from build123d import *

# Parameters (mm, degrees)
SKETCH1_W               = 75
SKETCH1_H               = 90
SKETCH1_W_2             = 50
SKETCH1_H_2             = 13
BOSS_EXTRUDE1_DEPTH     = 8
SKETCH2_R               = 18
SKETCH2_R_2             = 16
BOSS_EXTRUDE2_DEPTH     = 5
SKETCH3_R               = 2
CUT_EXTRUDE2_DEPTH      = 6
CUT_EXTRUDE2_DEPTH_BACK = 9
FILLET2_R               = 10
FILLET3_R               = 10
FILLET4_R               = 10
CUT_EXTRUDE3_REACH      = 10
SKETCH5_R               = 2.5
SKETCH7_W               = 5
SKETCH7_H               = 34
BOSS_EXTRUDE3_DEPTH     = 63
FILLET5_R               = 5
FILLET6_R               = 5
FILLET7_R               = 5
CUT_EXTRUDE4_REACH      = 92
CUT_EXTRUDE5_REACH      = 44
SKETCH14_R              = 2.5
SKETCH14_R_2            = 4


with BuildPart() as part:
    # Sketch1 → Boss-Extrude1 (new body)
    with BuildSketch(Plane(origin=(0, 0, 0), x_dir=(1, 0, 0), z_dir=(0, 1, 0))):
        with Locations((37.5, -45)):
            Rectangle(SKETCH1_W, SKETCH1_H)
        with Locations((100, -83.5)):
            Rectangle(SKETCH1_W_2, SKETCH1_H_2)
    extrude(amount=BOSS_EXTRUDE1_DEPTH)

    # Sketch2 → Boss-Extrude2 (add)
    with BuildSketch(Plane.XZ):
        with Locations((37.5, 45)):
            Circle(SKETCH2_R)
        with Locations((37.5, 45)):
            Circle(SKETCH2_R_2, mode=Mode.SUBTRACT)
    extrude(amount=BOSS_EXTRUDE2_DEPTH)

    # Sketch3 → Cut-Extrude2 (cut, two sides)
    with BuildSketch(Plane.XZ) as cut_extrude2_sk:
        with Locations((8.5, 74)):
            Circle(SKETCH3_R)
        with Locations((66.5, 74)):
            Circle(SKETCH3_R)
        with Locations((8.5, 16)):
            Circle(SKETCH3_R)
        with Locations((66.5, 16)):
            Circle(SKETCH3_R)
    extrude(amount=CUT_EXTRUDE2_DEPTH, mode=Mode.SUBTRACT)
    extrude(cut_extrude2_sk.sketch, amount=-CUT_EXTRUDE2_DEPTH_BACK, mode=Mode.SUBTRACT)

    # Fillet2
    fillet2_edges = [part.edges().sort_by_distance(p)[0] for p in [
        (0, 4, 0),
    ]]
    fillet(fillet2_edges, radius=FILLET2_R)

    # Fillet3
    fillet3_edges = [part.edges().sort_by_distance(p)[0] for p in [
        (0, 4, 90),
    ]]
    fillet(fillet3_edges, radius=FILLET3_R)

    # Fillet4
    fillet4_edges = [part.edges().sort_by_distance(p)[0] for p in [
        (75, 4, 0),
    ]]
    fillet(fillet4_edges, radius=FILLET4_R)

    # Sketch5 → Cut-Extrude3 (cut, up to next)
    with BuildSketch(Plane.XZ, mode=Mode.PRIVATE) as cut_extrude3_sk1:
        with Locations((55, 6)):
            Circle(SKETCH5_R)
    cut_extrude3_tool1 = extrude(cut_extrude3_sk1.sketch, amount=-CUT_EXTRUDE3_REACH, mode=Mode.PRIVATE) & part.part
    add(cut_extrude3_tool1.solids().sort_by_distance((55, 0, 6))[0], mode=Mode.SUBTRACT)
    # Sketch5 → Cut-Extrude3 (cut, up to next)
    with BuildSketch(Plane.XZ, mode=Mode.PRIVATE) as cut_extrude3_sk2:
        with Locations((20, 84)):
            Circle(SKETCH5_R)
    cut_extrude3_tool2 = extrude(cut_extrude3_sk2.sketch, amount=-CUT_EXTRUDE3_REACH, mode=Mode.PRIVATE) & part.part
    add(cut_extrude3_tool2.solids().sort_by_distance((20, 0, 84))[0], mode=Mode.SUBTRACT)
    # Sketch5 → Cut-Extrude3 (cut, up to next)
    with BuildSketch(Plane.XZ, mode=Mode.PRIVATE) as cut_extrude3_sk3:
        with Locations((55, 84)):
            Circle(SKETCH5_R)
    cut_extrude3_tool3 = extrude(cut_extrude3_sk3.sketch, amount=-CUT_EXTRUDE3_REACH, mode=Mode.PRIVATE) & part.part
    add(cut_extrude3_tool3.solids().sort_by_distance((55, 0, 84))[0], mode=Mode.SUBTRACT)
    # Sketch5 → Cut-Extrude3 (cut, up to next)
    with BuildSketch(Plane.XZ, mode=Mode.PRIVATE) as cut_extrude3_sk4:
        with Locations((20, 6)):
            Circle(SKETCH5_R)
    cut_extrude3_tool4 = extrude(cut_extrude3_sk4.sketch, amount=-CUT_EXTRUDE3_REACH, mode=Mode.PRIVATE) & part.part
    add(cut_extrude3_tool4.solids().sort_by_distance((20, 0, 6))[0], mode=Mode.SUBTRACT)

    # Sketch7 → Boss-Extrude3 (add)
    with BuildSketch(Plane(origin=(125, 0, 0), x_dir=(0, 0, -1), z_dir=(1, 0, 0))):
        with Locations((-87.5, 25)):
            Rectangle(SKETCH7_W, SKETCH7_H)
    extrude(amount=-BOSS_EXTRUDE3_DEPTH)

    # Fillet5
    fillet5_edges = [part.edges().sort_by_distance(p)[0] for p in [
        (125, 42, 87.5),
    ]]
    fillet(fillet5_edges, radius=FILLET5_R)

    # Fillet6
    fillet6_edges = [part.edges().sort_by_distance(p)[0] for p in [
        (125, 4, 77),
    ]]
    fillet(fillet6_edges, radius=FILLET6_R)

    # Fillet7
    fillet7_edges = [part.edges().sort_by_distance(p)[0] for p in [
        (62, 42, 87.5),
    ]]
    fillet(fillet7_edges, radius=FILLET7_R)

    # Sketch12 → Cut-Extrude4 (cut, up to next)
    with BuildSketch(Plane.XY.offset(90), mode=Mode.PRIVATE) as cut_extrude4_sk1:
        with BuildLine():
            Line((77.5, 26.5), (87.5, 26.5))
            ThreePointArc((87.5, 26.5), (91.5, 22.5), (87.5, 18.5))
            Line((87.5, 18.5), (77.5, 18.5))
            ThreePointArc((77.5, 18.5), (73.5, 22.5), (77.5, 26.5))
        make_face()
    cut_extrude4_tool1 = extrude(cut_extrude4_sk1.sketch, amount=-CUT_EXTRUDE4_REACH, mode=Mode.PRIVATE) & part.part
    add(cut_extrude4_tool1.solids().sort_by_distance((82.5, 22.5, 90))[0], mode=Mode.SUBTRACT)
    # Sketch12 → Cut-Extrude4 (cut, up to next)
    with BuildSketch(Plane.XY.offset(90), mode=Mode.PRIVATE) as cut_extrude4_sk2:
        with BuildLine():
            Line((70.5, 33), (79.5, 33))
            ThreePointArc((79.5, 33), (81, 31.5), (79.5, 30))
            Line((79.5, 30), (70.5, 30))
            ThreePointArc((70.5, 30), (69, 31.5), (70.5, 33))
        make_face()
    cut_extrude4_tool2 = extrude(cut_extrude4_sk2.sketch, amount=-CUT_EXTRUDE4_REACH, mode=Mode.PRIVATE) & part.part
    add(cut_extrude4_tool2.solids().sort_by_distance((75, 31.5, 90))[0], mode=Mode.SUBTRACT)
    # Sketch12 → Cut-Extrude4 (cut, up to next)
    with BuildSketch(Plane.XY.offset(90), mode=Mode.PRIVATE) as cut_extrude4_sk3:
        with BuildLine():
            Line((70.5, 12), (79.5, 12))
            ThreePointArc((79.5, 12), (81, 13.5), (79.5, 15))
            Line((79.5, 15), (70.5, 15))
            ThreePointArc((70.5, 15), (69, 13.5), (70.5, 12))
        make_face()
    cut_extrude4_tool3 = extrude(cut_extrude4_sk3.sketch, amount=-CUT_EXTRUDE4_REACH, mode=Mode.PRIVATE) & part.part
    add(cut_extrude4_tool3.solids().sort_by_distance((75, 13.5, 90))[0], mode=Mode.SUBTRACT)
    # Sketch12 → Cut-Extrude4 (cut, up to next)
    with BuildSketch(Plane.XY.offset(90), mode=Mode.PRIVATE) as cut_extrude4_sk4:
        with BuildLine():
            Line((103.5, 33), (112.5, 33))
            ThreePointArc((112.5, 33), (114, 31.5), (112.5, 30))
            Line((112.5, 30), (103.5, 30))
            ThreePointArc((103.5, 30), (102, 31.5), (103.5, 33))
        make_face()
    cut_extrude4_tool4 = extrude(cut_extrude4_sk4.sketch, amount=-CUT_EXTRUDE4_REACH, mode=Mode.PRIVATE) & part.part
    add(cut_extrude4_tool4.solids().sort_by_distance((108, 31.5, 90))[0], mode=Mode.SUBTRACT)
    # Sketch12 → Cut-Extrude4 (cut, up to next)
    with BuildSketch(Plane.XY.offset(90), mode=Mode.PRIVATE) as cut_extrude4_sk5:
        with BuildLine():
            Line((103.5, 12), (112.5, 12))
            ThreePointArc((112.5, 12), (114, 13.5), (112.5, 15))
            Line((112.5, 15), (103.5, 15))
            ThreePointArc((103.5, 15), (102, 13.5), (103.5, 12))
        make_face()
    cut_extrude4_tool5 = extrude(cut_extrude4_sk5.sketch, amount=-CUT_EXTRUDE4_REACH, mode=Mode.PRIVATE) & part.part
    add(cut_extrude4_tool5.solids().sort_by_distance((108, 13.5, 90))[0], mode=Mode.SUBTRACT)

    # Sketch14 → Cut-Extrude5 (cut, up to next)
    with BuildSketch(Plane.XZ, mode=Mode.PRIVATE) as cut_extrude5_sk1:
        with Locations((37.5, 57)):
            Circle(SKETCH14_R)
    cut_extrude5_tool1 = extrude(cut_extrude5_sk1.sketch, amount=-CUT_EXTRUDE5_REACH, mode=Mode.PRIVATE) & part.part
    add(cut_extrude5_tool1.solids().sort_by_distance((37.5, 0, 57))[0], mode=Mode.SUBTRACT)
    # Sketch14 → Cut-Extrude5 (cut, up to next)
    with BuildSketch(Plane.XZ, mode=Mode.PRIVATE) as cut_extrude5_sk2:
        with Locations((37.5, 45)):
            Circle(SKETCH14_R_2)
    cut_extrude5_tool2 = extrude(cut_extrude5_sk2.sketch, amount=-CUT_EXTRUDE5_REACH, mode=Mode.PRIVATE) & part.part
    add(cut_extrude5_tool2.solids().sort_by_distance((37.5, 0, 45))[0], mode=Mode.SUBTRACT)
    # Sketch14 → Cut-Extrude5 (cut, up to next)
    with BuildSketch(Plane.XZ, mode=Mode.PRIVATE) as cut_extrude5_sk3:
        with Locations((49.5, 45)):
            Circle(SKETCH14_R)
    cut_extrude5_tool3 = extrude(cut_extrude5_sk3.sketch, amount=-CUT_EXTRUDE5_REACH, mode=Mode.PRIVATE) & part.part
    add(cut_extrude5_tool3.solids().sort_by_distance((49.5, 0, 45))[0], mode=Mode.SUBTRACT)
    # Sketch14 → Cut-Extrude5 (cut, up to next)
    with BuildSketch(Plane.XZ, mode=Mode.PRIVATE) as cut_extrude5_sk4:
        with Locations((37.5, 33)):
            Circle(SKETCH14_R)
    cut_extrude5_tool4 = extrude(cut_extrude5_sk4.sketch, amount=-CUT_EXTRUDE5_REACH, mode=Mode.PRIVATE) & part.part
    add(cut_extrude5_tool4.solids().sort_by_distance((37.5, 0, 33))[0], mode=Mode.SUBTRACT)
    # Sketch14 → Cut-Extrude5 (cut, up to next)
    with BuildSketch(Plane.XZ, mode=Mode.PRIVATE) as cut_extrude5_sk5:
        with Locations((25.5, 45)):
            Circle(SKETCH14_R)
    cut_extrude5_tool5 = extrude(cut_extrude5_sk5.sketch, amount=-CUT_EXTRUDE5_REACH, mode=Mode.PRIVATE) & part.part
    add(cut_extrude5_tool5.solids().sort_by_distance((25.5, 0, 45))[0], mode=Mode.SUBTRACT)


solid = part.part
Here's how the part is built. I have some questions about the finished solid (model axes, mm). A direction names the side the tool comes from. Coordinates: 2 decimals unless noted, no trailing zeros. Loops run counter-clockwise (first coordinate to the right, second up) from the corner with the lowest first, then second, coordinate; pieces in that order, holes last. Notation, with made-up numbers: (-10, 47) -> (22, 47) arc R25 ccw to (22, 59) -> close; hole circle Ø2 at (87, -4.5). An arc over 180 degrees is marked (long way). Use one line per item in the form item = value. Start each with the question number.
(1) If we section it at B-B (x = 109.5): Please give me the cut outline in (y, z), then the cut area to 3 significant figures.
(2) If we section it at D-D (y = 4): Give the number of separate pieces and of enclosed holes in the cut face, then the cut area to 3 significant figures.
(3) Please list where these lines run through material, in increasing order: line 1 along Z through (x, y) = (66, 2); line 2 along Z through (x, y) = (66.5, 4.5); line 3 along Y through (x, z) = (66.5, 57).
(4) If we section it at A-A (z = 45): Please give me the cut outline in (x, y), then the cut area to 3 significant figures.
(5) On a 3-axis mill with a long thin cutter (end or side, diameter ignored), from which of +Z, -Z, +X, -X, +Y, -Y can I reach the whole of each face in a straight line? I mean faces 5 (the face through (66.24, 3.944, 17.983)), 6 (the face through (97, 4, 77)), 7 (the face through (83, 18.5, 88)), 8 (the face through (54.669, -2.465, 50.407)). Say none if no direction works.
(6) We'd pull the mould along Y, two halves only. Please class faces 1 (the face through (34, 0, 64)), 2 (the face through (114, 31.5, 87.5)), 3 (the face through (39, 4, 35)), 4 (the face through (108, 33, 88)): pulls with the +Y half, pulls with the -Y half, needs draft (parallel to the pull), parting line crosses it, or undercut.
(7) If we section it at C-C (y = 22.5): Please give me the cut outline in (x, z).
(8) Will these pins go through, and if not, where does the flat tip stop? pin 1 (8 mm diameter, centred on x = 40.5, z = 62, fed in from +Y); pin 2 (5 mm diameter, centred on x = 66.5, z = 16, fed in from -Y).
Verdict:
q1.outline = (0, 77) -> (8, 77) -> (8, 85) -> (12, 85) -> (12, 90) -> (0, 90) -> close; (15, 85) -> (30, 85) -> (30, 90) -> (15, 90) -> close; (33, 85) -> (42, 85) -> (42, 90) -> (33, 90) -> close
q1.area = 244 mm²
q2.separate_pieces = 1
q2.enclosed_holes = 13
q2.area = 7,070 mm²
q3.line_1 = 0.05 to 14.06, 17.94 to 72.06, 75.94 to 90
q3.line_2 = 0.11 to 14, 18 to 72, 76 to 90
q3.line_3 = 0 to 8
q4.outline = (0, 0) -> (19.5, 0) -> (19.5, -5) -> (21.5, -5) -> (21.5, 0) -> (23, 0) -> (23, 8) -> (0, 8) -> close; (28, 0) -> (33.5, 0) -> (33.5, 8) -> (28, 8) -> close; (41.5, 0) -> (47, 0) -> (47, 8) -> (41.5, 8) -> close; (52, 0) -> (53.5, 0) -> (53.5, -5) -> (55.5, -5) -> (55.5, 0) -> (75, 0) -> (75, 8) -> (52, 8) -> close
q4.area = 476 mm²
q5.face_5 = +Y, -Y
q5.face_6 = -Z, +X, +Y, -Y
q5.face_7 = +Z, -Z
q5.face_8 = -Y
q6.face_1 = pulls with the -Y half
q6.face_2 = undercut
q6.face_3 = needs draft
q6.face_4 = undercut
q7.outline = (62, 85) -> (73.5, 85) -> (73.5, 90) -> (62, 90) -> close; (91.5, 85) -> (125, 85) -> (125, 90) -> (91.5, 90) -> close
q8.pin_1 = 8
q8.pin_2 = 0
